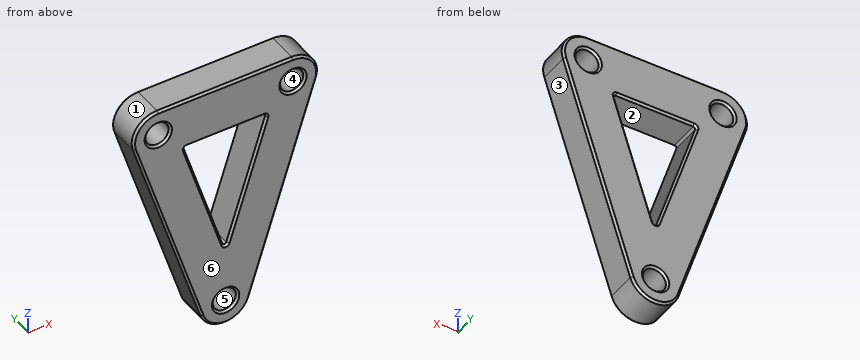
from build123d import *

# Parameters (mm, degrees)
SKETCH1_R           = 2.1828125
BOSS_EXTRUDE2_DEPTH = 6.35
CHAMFER2_SIZE       = 0.396875


with BuildPart() as part:
    # Sketch1 → Boss-Extrude2 (new body)
    with BuildSketch(Plane(origin=(0, 0, 0), x_dir=(1, 0, 0), z_dir=(0, 1, 0))):
        with BuildLine():
            Line((-4.535244397, 1.453603973), (-17.235244397, -38.170396027))
            ThreePointArc((-17.235244397, -38.170396027), (-16.547349423, -42.431010628), (-12.7, -44.3865))
            Line((-12.7, -44.3865), (12.7, -44.3865))
            ThreePointArc((12.7, -44.3865), (16.547349423, -42.431010628), (17.235244397, -38.170396027))
            Line((17.235244397, -38.170396027), (4.535244397, 1.453603973))
            ThreePointArc((4.535244397, 1.453603973), (0, 4.7625), (-4.535244397, 1.453603973))
        make_face()
        Circle(SKETCH1_R, mode=Mode.SUBTRACT)
        with Locations((12.7, -39.624)):
            Circle(SKETCH1_R, mode=Mode.SUBTRACT)
        with Locations((-12.7, -39.624)):
            Circle(SKETCH1_R, mode=Mode.SUBTRACT)
        with BuildLine():
            Line((-0.377937033, -11.581541204), (-7.67343387, -34.343491336))
            ThreePointArc((-7.67343387, -34.343491336), (-7.616109289, -34.698542552), (-7.295496837, -34.8615))
            Line((-7.295496837, -34.8615), (7.295496837, -34.8615))
            ThreePointArc((7.295496837, -34.8615), (7.616109289, -34.698542552), (7.67343387, -34.343491336))
            Line((7.67343387, -34.343491336), (0.377937033, -11.581541204))
            ThreePointArc((0.377937033, -11.581541204), (0, -11.305799869), (-0.377937033, -11.581541204))
        make_face(mode=Mode.SUBTRACT)
    extrude(amount=BOSS_EXTRUDE2_DEPTH)

    # Chamfer2
    chamfer2_edges = [part.edges().sort_by_distance(p)[0] for p in [
        (-16.547349423, 6.35, 42.431010628),
        (0, 6.35, 44.3865),
        (-2.1828125, 0, 0),
        (-2.1828125, 6.35, 0),
        (10.5171875, 0, 39.624),
        (16.547349423, 6.35, 42.431010628),
        (10.5171875, 6.35, 39.624),
        (-14.8828125, 0, 39.624),
        (10.885244397, 6.35, 18.358396027),
        (-14.8828125, 6.35, 39.624),
        (7.616109289, 0, 34.698542552),
        (4.025685452, 0, 22.96251627),
        (0, 0, 11.305799869),
        (-4.025685452, 0, 22.96251627),
        (-7.616109289, 0, 34.698542552),
        (0, 0, 34.8615),
        (7.616109289, 6.35, 34.698542552),
        (4.025685452, 6.35, 22.96251627),
        (0, 6.35, 11.305799869),
        (-4.025685452, 6.35, 22.96251627),
        (-7.616109289, 6.35, 34.698542552),
        (0, 6.35, 34.8615),
        (0, 6.35, -4.7625),
        (10.885244397, 0, 18.358396027),
        (16.547349423, 0, 42.431010628),
        (0, 0, 44.3865),
        (-16.547349423, 0, 42.431010628),
        (-10.885244397, 0, 18.358396027),
        (0, 0, -4.7625),
        (-10.885244397, 6.35, 18.358396027),
    ]]
    chamfer(chamfer2_edges, length=CHAMFER2_SIZE)


solid = part.part
The model under review builds one solid part; all positions refer to its coordinate system, in mm. Face numbers are marked on the shaded views. A direction names the side the tool comes from. Give positions to 0.01 mm unless a question says otherwise; leave off trailing zeros. Loops run counter-clockwise (first coordinate to the right, second up) from the corner with the lowest first, then second, coordinate; pieces in that order, holes last. Notation, with made-up numbers: (10.25, -32.75) -> (34.25, -32.75) arc R15 cw to (34.25, -27.75) -> close; hole circle Ø6 at (56, 7.25). An arc over 180 degrees is marked (long way). Put each result on its own line as item: value. Start each with the question number.
1. We need section C-C on x = 5.5. State the section outline as (y, z) points.
2. For the marked faces 1 and 2, list the 3-axis set-ups (+Z, -Z, +X, -X, +Y, -Y) from which the entire face can be reached by the end or side of a thin tool; tool diameter is ignored.
3. We need section A-A on z = 22. State the section outline as (x, y) points, then the cut area to 3 significant figures.
4. We need section B-B on y = 3.75. State the section outline as (x, z) points (1 decimal).
5. Clearance check with flat-ended pins moving along their axes: P1, Ø1.7, axis at x = -3.5, y = 2, coming from the -Z side; P2, Ø5.5, axis at x = 0, z = 0, coming from the -Y side; P3, Ø4, axis at x = 12.7, z = 39.624, coming from the -Y side. State where each tip first meets the part, or that it passes through.
6. Wall thickness on probe 1 along Z at (x, y) = (0, 4.3); probe 2 along X at (y, z) = (4.25, 40.5); probe 3 along X at (y, z) = (3.5, 26.5): over which ranges is each line inside the solid? List them lowest first.
7. We need section D-D on z = 4.5. State the section outline as (x, y) points, then the cut area to 3 significant figures.
8. Mouldability with a two-part tool opening along Z and no side actions: class the marked faces 3, 4, 5 and 6 as released by +Z, released by -Z, zero draft, split by the parting line, or undercut.
Determined:
1. outline: (0, 2.86) -> (0.4, 1.56) -> (5.95, 1.56) -> (6.35, 2.86) -> (6.35, 26.26) -> (5.95, 27.56) -> (0.4, 27.56) -> (0, 26.26) -> close; (0, 35.26) -> (0.4, 34.86) -> (5.95, 34.86) -> (6.35, 35.26) -> (6.35, 43.99) -> (5.95, 44.39) -> (0.4, 44.39) -> (0, 43.99) -> close
2. face 1: -X, +Y, -Y
2. face 2: +Y, -Y
3. outline: (-12.05, 0.4) -> (-11.64, 0) -> (-4.13, 0) -> (-3.72, 0.4) -> (-3.72, 5.95) -> (-4.13, 6.35) -> (-11.64, 6.35) -> (-12.05, 5.95) -> close; (3.72, 0.4) -> (4.13, 0) -> (11.64, 0) -> (12.05, 0.4) -> (12.05, 5.95) -> (11.64, 6.35) -> (4.13, 6.35) -> (3.72, 5.95) -> close
3. area: 105 mm^2
4. outline: (-17.2, 38.2) -> (-4.5, -1.5) arc R4.8 ccw to (4.5, -1.5) -> (17.2, 38.2) arc R4.8 ccw to (12.7, 44.4) -> (-12.7, 44.4) arc R4.8 ccw to start; hole circle Ø4.4 at (-12.7, 39.6); hole (-7.7, 34.3) -> (-0.4, 11.6) arc R0.4 ccw to (0.4, 11.6) -> (7.7, 34.3) arc R0.4 ccw to (7.3, 34.9) -> (-7.3, 34.9) arc R0.4 ccw to start; hole circle Ø4.4 at (0, 0); hole circle Ø4.4 at (12.7, 39.6)
5. P1: z = -3.96
5. P2: y = 0
5. P3: through
6. probe 1: -4.76 to -2.18, 2.18 to 11.31, 34.86 to 44.39
6. probe 2: -17.38 to -14.7, -10.7 to 10.7, 14.7 to 17.38
6. probe 3: -13.49 to -5.16, 5.16 to 13.49
7. outline: (-6.44, 0.4) -> (-6.03, 0) -> (6.03, 0) -> (6.44, 0.4) -> (6.44, 5.95) -> (6.03, 6.35) -> (-6.03, 6.35) -> (-6.44, 5.95) -> close
7. area: 81.5 mm^2
8. face 3: released by -Z
8. face 4: undercut
8. face 5: undercut
8. face 6: zero draft
